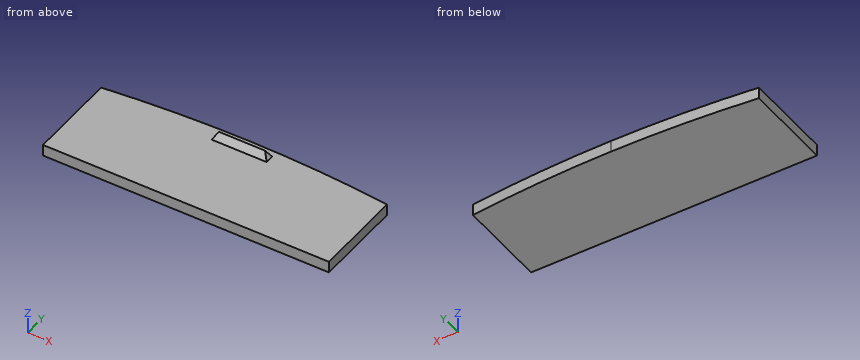
from build123d import *

# Parameters (mm, degrees)
BOSS_EXTRU_2_DEPTH = 4
ESQUISSE6_W        = 19.024162062
ESQUISSE6_H        = 3
BOSS_EXTRU_3_DEPTH = 3
BOSS_EXTRU_3_TAPER = 30


with BuildPart() as part:
    # Esquisse2 → Boss.-Extru.2 (new body)
    with BuildSketch(Plane.XY):
        with BuildLine():
            Line((15.843049481, 153.91195697), (15.843049481, 122.649102361))
            Line((15.843049481, 122.649102361), (114.867211543, 122.649102361))
            Line((114.867211543, 122.649102361), (114.867211543, 153.891733148))
            ThreePointArc((114.867211543, 153.891733148), (90.104041762, 155.959238078), (65.264290885, 156.649115353))
            ThreePointArc((65.264290885, 156.649115353), (40.515800335, 155.964301811), (15.843049481, 153.91195697))
        make_face()
    extrude(amount=BOSS_EXTRU_2_DEPTH)

    # Esquisse6 → Boss.-Extru.3 (add)
    with BuildSketch(Plane.XY.offset(4)):
        with Locations((65.355130512, 152.77778229)):
            Rectangle(ESQUISSE6_W, ESQUISSE6_H)
    extrude(amount=BOSS_EXTRU_3_DEPTH, taper=BOSS_EXTRU_3_TAPER)


solid = part.part
Input: part model. Units: mm. Frame: model coordinates. Give positions to 0.01 mm unless a question says otherwise; leave off trailing zeros. Order: outer loops, then holes, each group sorted by start corner. A loop starts at its lowest first (then second) coordinate and runs counter-clockwise, first axis right, second up. Notation, with made-up numbers: (-2, 80) - (4, 80) arc R19 ccw to (4, 85) - close; hole circle Ø11 at (89, 58). An arc over 180 degrees is marked (long way). Write each question's results on one line, items separated by ' | '.
Item 1: Section C-C (x = 96.5). Return loops of the section in (y, z), and give its area (3 significant figures).
A:
outline: (122.65, 0) - (155.56, 0) - (155.56, 4) - (122.65, 4) - close | area: 132 mm^2
Item 2: Section A-A (z = 3). Return loops of the section in (x, y).
A:
outline: (15.84, 122.65) - (114.87, 122.65) - (114.87, 153.89) arc R447.54 ccw to (15.84, 153.91) - close
Item 3: Material intervals for line 1 along Z through (x, y) = (58.5, 149.5); line 2 along Y through (x, z) = (100.5, 3.75); line 3 along Y through (x, z) = (60.5, 0.5), sorted ascending.
A:
line 1: z = 0 to 4 | line 2: y = 122.65 to 155.26 | line 3: y = 122.65 to 156.62
Item 4: Contact query for flat-ended pins moving along their axis: pin 1 Ø3 at (x, y) = (40, 150.5) entering from +Z; pin 2 Ø6 at (x, y) = (94.5, 127) entering from -Z. Output: stop coordinate, or through.
A:
pin 1: stops at z = 4 | pin 2: stops at z = 0
Item 5: Section B-B (y = 144.5). Return loops of the section in (x, z).
A:
outline: (15.84, 0) - (114.87, 0) - (114.87, 4) - (15.84, 4) - close
